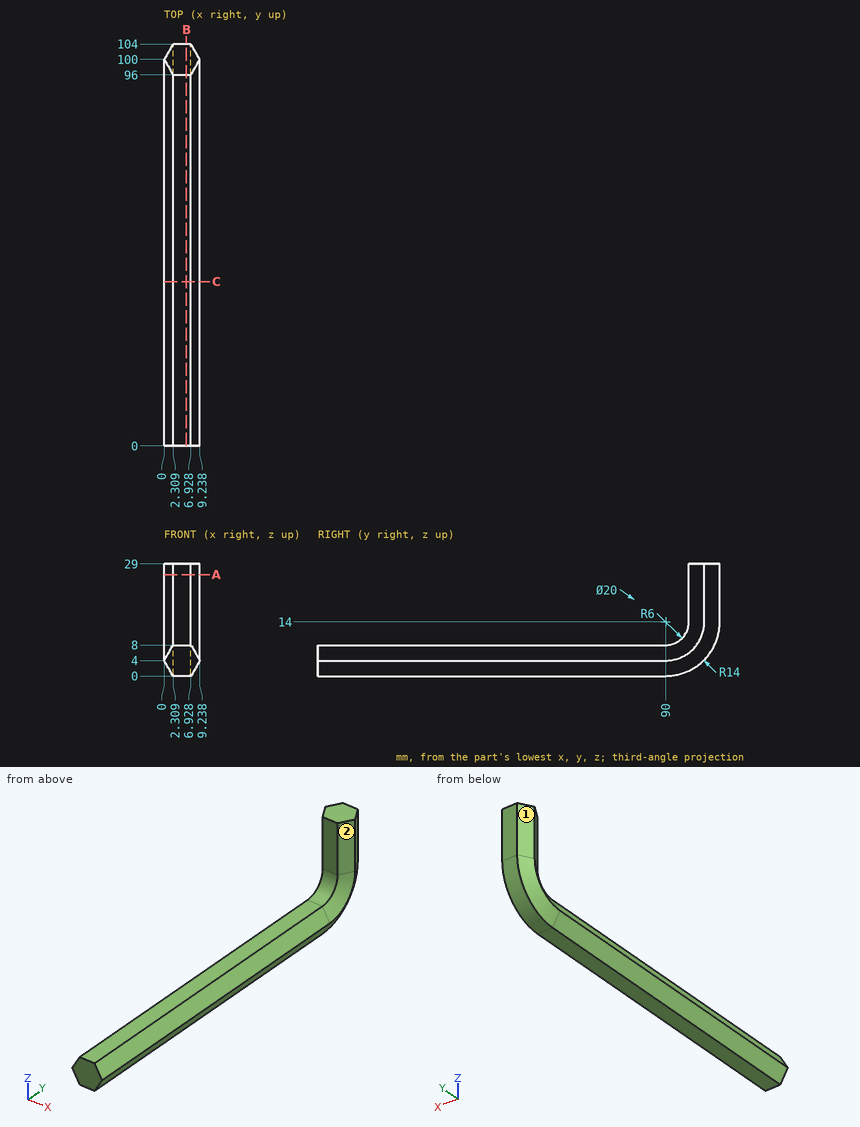
Verification items for this drawing (mm, ordinates from the low corner). A direction names the side the tool comes from. Give positions to 0.01 mm unless a question says otherwise; leave off trailing zeros. Write each loop counter-clockwise with the first axis right and the second up, starting at its lowest first coordinate (ties: lowest second). Pieces come first, ordered by that corner, then holes. Notation, with made-up numbers: (69.25, -20.5) - (92.25, -20.5) arc R34 ccw to (92.25, 13.5) - close; hole circle Ø5 at (54, 22). An arc over 180 degrees is marked (long way). Answer as a JSON object with one key per item and string values. Group by question number.
1) Sectioned sample at A-A (z = 26.25). Record the cut outline in (x, y), then the cut area to 3 significant figures.
2) Thickness scan on probe 1 along Z at (x, y) = (2.5, 56.5); probe 2 along Y at (x, z) = (5.25, 25.5); probe 3 along Y at (x, z) = (3, 1.5) (1 decimal). Record the ranges inside material, lowest first. Write a range as from..to.
3) Access from +Z, -Z, +X, -X, +Y, -Y to the whole of each face (thin tool, end or side, straight path). Record for the marked faces 1 and 2.
4) Depth check by flat-ended pin: P1, Ø1.5, axis at y = 84.5, z = 5.5, coming from the -X side; P2, Ø2, axis at x = 3.5, y = 80.5, coming from the +Z side; P3, Ø1.5, axis at x = 8, z = 25.5, coming from the -Y side (1 decimal). Enter the tip coordinate at first touch or a pass-through.
5) Sectioned sample at B-B (x = 5.75). Record the cut outline in (y, z).
6) Sectioned sample at C-C (y = 42.5). Record the cut outline in (x, z), then the cut area to 3 significant figures.
Geometry results:
{
 "1": {"outline": "(0, 100) - (2.31, 96) - (6.93, 96) - (9.24, 100) - (6.93, 104) - (2.31, 104) - close", "area": "55.4 mm^2"},
 "2": {"probe 1": "z = 0..8", "probe 2": "y = 96..104", "probe 3": "y = 0..96.3"},
 "3": {"face 1": "+Z, -Z, -X, +Y", "face 2": "+Z, +X, -Y"},
 "4": {"P1": "stops at x = 0.43", "P2": "stops at z = 8", "P3": "stops at y = 96.6"},
 "5": {"outline": "(0, 0) - (90, 0) arc R14 ccw to (104, 14) - (104, 29) - (96, 29) - (96, 14) arc R6 cw to (90, 8) - (0, 8) - close"},
 "6": {"outline": "(0, 4) - (2.31, 0) - (6.93, 0) - (9.24, 4) - (6.93, 8) - (2.31, 8) - close", "area": "55.4 mm^2"}
}
